```python
from build123d import *

# Parameters (mm, degrees)
SKETCH_W   = 45.3
SKETCH_H   = 22
SKETCH_W_2 = 5.1
SKETCH_H_2 = 13
PAD_DEPTH  = 13
FILLET_R   = 4


with BuildPart() as part:
    # Sketch → Pad (new body)
    with BuildSketch(Plane.XY):
        Rectangle(SKETCH_W, SKETCH_H)
        Rectangle(SKETCH_W_2, SKETCH_H_2, mode=Mode.SUBTRACT)
        with Locations((-15.1, 0)):
            Rectangle(SKETCH_W_2, SKETCH_H_2, mode=Mode.SUBTRACT)
        with Locations((15.1, 0)):
            Rectangle(SKETCH_W_2, SKETCH_H_2, mode=Mode.SUBTRACT)
    extrude(amount=-PAD_DEPTH)

    # Fillet
    fillet_edges = [part.edges().sort_by_distance(p)[0] for p in [
        (-22.65, -11, -6.5),
        (22.65, -11, -6.5),
        (22.65, 11, -6.5),
        (-22.65, 11, -6.5),
    ]]
    fillet(fillet_edges, radius=FILLET_R)


solid = part.part
```
Check sheet for the modelled part. Datum: model origin and axes. Units: mm. A direction names the side the tool comes from. Coordinates: 2 decimals unless noted, no trailing zeros. Order: outer loops, then holes, each group sorted by start corner. A loop starts at its lowest first (then second) coordinate and runs counter-clockwise, first axis right, second up. Notation, with made-up numbers: M 51,89.25 L 96,89.25 A21 ccw 96,100.25 Z; hole C 23,25 d5. An arc over 180 degrees is marked long. One line per question, with ' | ' between items. Start each with the question number.
Item 1: Sectioned sample at C-C on z = -10. Record the cut outline in (x, y), and give its area (3 significant figures).
Item 2: Material ranges on line 1 (X direction, y = -5.5, z = -9); line 2 (Y direction, x = 14, z = -11.75); line 3 (X direction, y = -8.5, z = -8), recorded low to high.
Item 3: Gauge pin test, flat end, axial feed: P1, Ø1, axis at x = -2.5, y = 7.5, coming from the +Z side. Record the tip position at first contact, or that the pin passes through.
Item 4: Sectioned sample at B-B on x = -1.5. Record the cut outline in (y, z).
Item 5: Sectioned sample at D-D on y = 9.5. Record the cut outline in (x, z), and give its area (3 significant figures).
Item 6: Mould release check, pull along X, two halves, no side actions. Record for faces 1 (the flat face through (-15, 6.5, -6)), 2 (the cylindrical face through (21.447, -9.859, -6.591)), 3 (the flat face through (-5, 0, -13)): pulls with the +X half, pulls with the -X half, needs draft (parallel to the pull), parting line crosses it, or undercut.
Item 7: Access from +Z, -Z, +X, -X, +Y, -Y to the whole of each face (thin tool, end or side, straight path). Record for faces 4 (the cylindrical face through (-21.509, -9.797, -6.591)), 5 (the flat face through (-15, -6.5, -6)).
Item 8: Sectioned sample at A-A on y = 3.75. Record the cut outline in (x, z).
Answer below:
1) outline: M -22.65,-7 A4 ccw -18.65,-11 L 18.65,-11 A4 ccw 22.65,-7 L 22.65,7 A4 ccw 18.65,11 L -18.65,11 A4 ccw -22.65,7 Z; hole M -17.65,-6.5 L -12.55,-6.5 L -12.55,6.5 L -17.65,6.5 Z; hole M -2.55,-6.5 L 2.55,-6.5 L 2.55,6.5 L -2.55,6.5 Z; hole M 12.55,-6.5 L 17.65,-6.5 L 17.65,6.5 L 12.55,6.5 Z | area: 784 mm^2
2) line 1: x = -22.65 to -17.65, -12.55 to -2.55, 2.55 to 12.55, 17.65 to 22.65 | line 2: y = -11 to -6.5, 6.5 to 11 | line 3: x = -22.36 to 22.36
3) P1: stops at z = 0
4) outline: M -11,-13 L -6.5,-13 L -6.5,0 L -11,0 Z; M 6.5,-13 L 11,-13 L 11,0 L 6.5,0 Z
5) outline: M -21.77,-13 L 21.77,-13 L 21.77,0 L -21.77,0 Z | area: 566 mm^2
6) face 1: undercut | face 2: pulls with the +X half | face 3: needs draft
7) face 4: +Z, -Z, -X, -Y | face 5: +Z, -Z
8) outline: M -22.65,-13 L -17.65,-13 L -17.65,0 L -22.65,0 Z; M -12.55,-13 L -2.55,-13 L -2.55,0 L -12.55,0 Z; M 2.55,-13 L 12.55,-13 L 12.55,0 L 2.55,0 Z; M 17.65,-13 L 22.65,-13 L 22.65,0 L 17.65,0 Z
